```python
from build123d import *

# Parameters (mm, degrees)
F0_W            = 72.5
F0_H            = 50
F1_DEPTH        = 30
F2_R            = 16
F3_DEPTH        = 30.001
F5_D            = 6.1
F5_DEPTH        = 8
F5_TIP          = 1.832624888
F6_R            = 32.5
F7_DEPTH        = 15
F8_R            = 24.99999
F10_D           = 5.5
F10_CBORE_D     = 9.5
F10_CBORE_DEPTH = 5
F11_W           = 1.7334403427
F11_H           = 15
F12_DEPTH       = 50.001


# Not quite as in the source:
# - a fillet or chamfer is up to 0.001 mm smaller than in the source, because OpenCascade refuses the exact size


with BuildPart() as f1:
    # F0 (on Top) → F1 (new body)
    with BuildSketch(Plane.XY):
        with Locations((-18.75, 0)):
            Rectangle(F0_W, F0_H)
    extrude(amount=F1_DEPTH)

    # F2 (on face) → F3 (cut, through all)
    with BuildSketch(Plane.XY.offset(30)):
        with Locations((-30, 0)):
            Circle(F2_R)
    extrude(amount=-F3_DEPTH, mode=Mode.SUBTRACT)

    # F5
    with Locations(Plane.XY.offset(30)):
        with Locations((0, 0)):
            Hole(F5_D / 2, depth=F5_DEPTH)
            with Locations((0, 0, -(F5_DEPTH + F5_TIP / 2))):  # 118° drill point
                Cone(0, F5_D / 2, F5_TIP, mode=Mode.SUBTRACT)

    # F6 (on face) → F7 (cut)
    with BuildSketch(Plane(origin=(0, 0, 0), x_dir=(1, 0, 0), z_dir=(0, 0, -1))):
        with Locations((-30, 0)):
            Circle(F6_R)
    extrude(amount=-F7_DEPTH, mode=Mode.SUBTRACT)

    # F8 (radius 25 in the source; OpenCascade refuses exactly that, so slightly less here)
    f8_edges = [f1.edges().sort_by_distance(p)[0] for p in [
        (-55, -25, 15),
        (-55, 25, 15),
    ]]
    fillet(f8_edges, radius=F8_R)

    # F10 (through all)
    with Locations(Plane.XY.offset(30)):
        with Locations((7.5, 15), (7.5, -15)):
            CounterBoreHole(F10_D / 2, F10_CBORE_D / 2, F10_CBORE_DEPTH)

    # F11 (on face) → F12 (cut, through all)
    with BuildSketch(Plane(origin=(0, 25, 0), x_dir=(-1, 0, 0), z_dir=(0, 1, 0))):
        with Locations((8.3667201714, 7.5)):
            Rectangle(F11_W, F11_H)
    extrude(amount=-F12_DEPTH, mode=Mode.SUBTRACT)


solid = f1.part
```
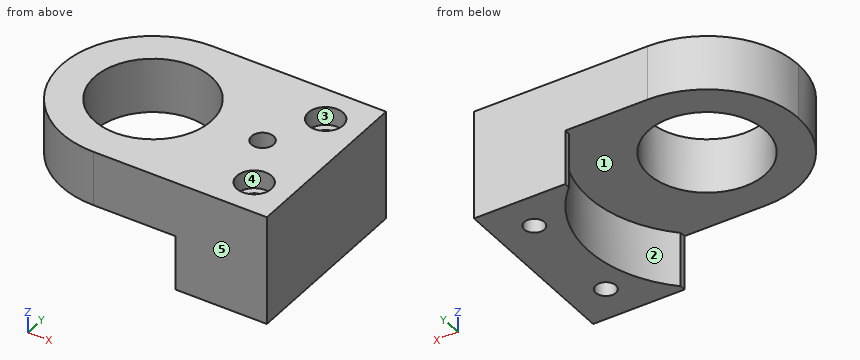
Design review of the part built by this model. Coordinates are the model's own, in mm. Face numbers are marked on the shaded views. A direction names the side the tool comes from. Coordinates: 2 decimals unless noted, no trailing zeros. Loops run counter-clockwise (first coordinate to the right, second up) from the corner with the lowest first, then second, coordinate; pieces in that order, holes last. Notation, with made-up numbers: (54.5, 59) - (76.5, 59) arc R29 cw to (76.5, 93) - close; hole circle Ø5 at (23.25, -26). An arc over 180 degrees is marked (long way). Use CSV: the item, a comma, the result in double quotes. Start each with the question number.
1) Consider section B-B on x = 7.5. Write out the cut boundary in (y, z).
2) The part is to be moulded in two halves that separate along X. For the marked faces 1, 2 and 3, say which applies: +X half, -X half, draft (parallel to the pull), parting line (faces both ways), or undercut.
3) For pin 1 Ø0.5 at (y, z) = (-24.5, 7) entering from -X; pin 2 Ø8 at (x, y) = (-34, -18.5) entering from -Z; pin 3 Ø5 at (x, y) = (0, 0) entering from +Z, all flat-tipped, find the tip position at first contact; note any pin that passes through.
4) Wall thickness on L1, parallel to Y at x = 7.5, z = 14.5; L2, parallel to Y at x = 7.5, z = 27.85; L3, parallel to Y at x = 0, z = 26: over which ranges is each line inside the solid? List them lowest first. Write a range as from..to.
5) Consider section A-A on z = 17.25. Give the number of separate pieces and of enclosed holes in the cut face, then the cut area to 3 significant figures.
6) Consider section D-D on y = 15. Write out the cut boundary in (x, z), then the cut area to 3 significant figures.
7) Tool access review of the marked faces 4 and 5: name each direction out of +Z, -Z, +X, -X, +Y, -Y from which nothing blocks a thin tool from reaching the whole face with its end or side.
Geometry says:
1,outline,"(-25, 0) - (-17.75, 0) - (-17.75, 25) - (-19.75, 25) - (-19.75, 30) - (-25, 30) - close; (-12.25, 0) - (12.25, 0) - (12.25, 25) - (10.25, 25) - (10.25, 30) - (-10.25, 30) - (-10.25, 25) - (-12.25, 25) - close; (17.75, 0) - (25, 0) - (25, 30) - (19.75, 30) - (19.75, 25) - (17.75, 25) - close"
2,face 1,"draft"
2,face 2,"-X half"
2,face 3,"undercut"
3,pin 1,"x = -7.5"
3,pin 2,"z = 15"
3,pin 3,"z = 21.67"
4,L1,"-25..-17.75, -12.25..12.25, 17.75..25"
4,L2,"-25..-19.75, -10.25..10.25, 19.75..25"
4,L3,"-25..-3.05, 3.05..25"
5,separate pieces,"1"
5,enclosed holes,"3"
5,area,"2,500 mm^2"
6,outline,"(-50, 15) - (-35.57, 15) - (-35.57, 30) - (-50, 30) - close; (-24.43, 15) - (-1.17, 15) - (-1.17, 0) - (4.75, 0) - (4.75, 25) - (2.75, 25) - (2.75, 30) - (-24.43, 30) - close; (10.25, 0) - (17.5, 0) - (17.5, 30) - (12.25, 30) - (12.25, 25) - (10.25, 25) - close"
6,area,"940 mm^2"
7,face 4,"+Z"
7,face 5,"+Z, -Z, +X, -X, -Y"
